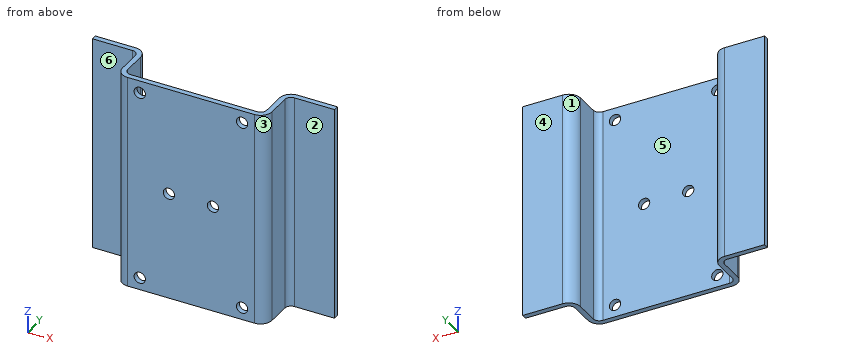
```python
from build123d import *

# Parameters (mm, degrees)
F1_DEPTH = 69.85
F2_R     = 3.69316
F3_R     = 1.98374
F4_R     = 1.8288
F5_DEPTH = 1.70942


with BuildPart() as f1:
    # F0 (on Top) → F1 (new body)
    with BuildSketch(Plane.XY):
        Polygon((0, -13.290575), (0, 0), (-16.70942, 0), (-16.70942, -1.70942), (-1.70942, -1.70942), (-1.70942, -14.999995), (46.79058, -14.999995), (46.79058, -1.70942), (61.79058, -1.70942), (61.79058, 0), (45.08116, 0), (45.08116, -13.290575), align=None)
    extrude(amount=F1_DEPTH)

    # F2
    f2_edges = [f1.edges().sort_by_distance(p)[0] for p in [
        (46.79058, -14.999995, 34.925),
        (-1.70942, -14.999995, 34.925),
        (0, 0, 34.925),
        (45.08116, 0, 34.925),
    ]]
    fillet(f2_edges, radius=F2_R)

    # F3
    f3_edges = [f1.edges().sort_by_distance(p)[0] for p in [
        (0, -13.290575, 34.925),
        (45.08116, -13.290575, 34.925),
        (46.79058, -1.70942, 34.925),
        (-1.70942, -1.70942, 34.925),
    ]]
    fillet(f3_edges, radius=F3_R)

    # F4 (on face) → F5 (cut, through all)
    with BuildSketch(Plane.XZ.offset(14.999995)):
        with Locations((39.12867, 65.88125)):
            Circle(F4_R)
        with Locations((5.95249, 65.88125)):
            Circle(F4_R)
        with Locations((5.95249, 3.96875)):
            Circle(F4_R)
        with Locations((39.12867, 3.96875)):
            Circle(F4_R)
        with Locations((15.39683, 34.925)):
            Circle(F4_R)
        with Locations((29.68433, 34.925)):
            Circle(F4_R)
    extrude(amount=-F5_DEPTH, mode=Mode.SUBTRACT)


solid = f1.part
```
Source: CAD feature listing. Evaluate the final solid. Frame: model axes, mm. Face numbers are marked on the shaded views. A direction names the side the tool comes from. Coordinates: 2 decimals unless noted, no trailing zeros. Loops run counter-clockwise (first coordinate to the right, second up) from the corner with the lowest first, then second, coordinate; pieces in that order, holes last. Notation, with made-up numbers: M 81,47.5 L 93,47.5 A24 ccw 93,75.5 Z; hole C 74,62.25 d8. An arc over 180 degrees is marked long. Use CSV: the item, a comma, the result in double quotes.
(1) Line query: line 1 (X direction, y = -10.25, z = 16.5); line 2 (Y direction, x = 28, z = 40.5); line 3 (Y direction, x = -12, z = 20.5). Output: solid intervals per line, ascending. Write a range as [from, to].
Answers follow:
line 1,"[-1.71, 0], [45.08, 46.79]"
line 2,"[-15, -13.29]"
line 3,"[-1.71, 0]"
(2) Contact query for flat-ended pins moving along their axis: pin 1 (4 mm diameter, centred on x = 39.13, z = 3.97, fed in from +Y); pin 2 (8.5 mm diameter, centred on y = -8, z = 32.5, fed in from -X); pin 3 (8.5 mm diameter, centred on y = -8, z = 39.5, fed in from +X). Output: stop coordinate, or through.
Answers follow:
pin 1,"y = -13.29"
pin 2,"x = -1.71"
pin 3,"x = 46.79"
(3) Cut plane C-C on z = 59.5. Return loops of the section in (x, y), and give its area (3 significant figures).
Answers follow:
outline,"M -16.71,-1.71 L -3.69,-1.71 A1.98 cw -1.71,-3.69 L -1.71,-11.31 A3.69 ccw 1.98,-15 L 43.1,-15 A3.69 ccw 46.79,-11.31 L 46.79,-3.69 A1.98 cw 48.77,-1.71 L 61.79,-1.71 L 61.79,0 L 48.77,0 A3.69 ccw 45.08,-3.69 L 45.08,-11.31 A1.98 cw 43.1,-13.29 L 1.98,-13.29 A1.98 cw 0,-11.31 L 0,-3.69 A3.69 ccw -3.69,0 L -16.71,0 Z"
area,"171 mm²"
(4) Cut plane A-A on y = -5.5. Return loops of the section in (x, z).
Answers follow:
outline,"M -1.71,0 L 0,0 L 0,69.85 L -1.71,69.85 Z; M 45.08,0 L 46.79,0 L 46.79,69.85 L 45.08,69.85 Z"
(5) Reachability of the marked faces 4, 5 and 6 from +Z, -Z, +X, -X, +Y, -Y: full face, straight path, thin tool, end or side. Return the list, or none.
Answers follow:
face 4,"+Z, -Z, +X, -X, +Y"
face 5,"+Z, -Z, +Y"
face 6,"+Z, -Z, -X, -Y"
(6) Draft query along X for the marked faces 1, 2 and 3. Return one class per face: pulls with the +X half, pulls with the -X half, needs draft (parallel to the pull), parting line crosses it, or undercut.
Answers follow:
face 1,"undercut"
face 2,"needs draft"
face 3,"pulls with the +X half"
(7) Cut plane B-B on x = 5.5. Return loops of the section in (y, z), and give its area (3 significant figures).
Answers follow:
outline,"M -15,0 L -13.29,0 L -13.29,2.2 L -15,2.2 Z; M -15,5.74 L -13.29,5.74 L -13.29,64.11 L -15,64.11 Z; M -15,67.65 L -13.29,67.65 L -13.29,69.85 L -15,69.85 Z"
area,"107 mm²"
